from build123d import *

# Parameters (mm, degrees)
SKETCH1_R           = 25
BOSS_EXTRUDE1_DEPTH = 60
SKETCH2_R           = 25
BOSS_EXTRUDE2_DEPTH = 120.5
CUT_EXTRUDE5_DEPTH  = 60
FILLET1_R           = 12


with BuildPart() as part:
    # Sketch1 → Boss-Extrude1 (new body)
    with BuildSketch(Plane.XY):
        with BuildLine():
            Line((60, 30), (200, 30))
            Line((200, 30), (200, -30))
            Line((200, -30), (60, -30))
            ThreePointArc((60, -30), (44.188611699, -32.565835097), (30, -40))
            ThreePointArc((30, -40), (-50, 0), (30, 40))
            ThreePointArc((30, 40), (44.188611699, 32.565835097), (60, 30))
        make_face()
        Circle(SKETCH1_R, mode=Mode.SUBTRACT)
    extrude(amount=BOSS_EXTRUDE1_DEPTH)

    # Sketch2 → Boss-Extrude2 (add)
    with BuildSketch(Plane(origin=(200, 0, 0), x_dir=(0, 0, -1), z_dir=(1, 0, 0))):
        with Locations((-30, 0)):
            Circle(SKETCH2_R)
    extrude(amount=BOSS_EXTRUDE2_DEPTH)

    # Sketch8 → Cut-Extrude5 (cut)
    with BuildSketch(Plane(origin=(200, 0, 0), x_dir=(0, 0, -1), z_dir=(1, 0, 0))):
        Polygon((-60, 11.94), (-41.94, 30), (-60, 30), align=None)
        Polygon((0, 30), (-16.229667357, 30), (0, 11.94), align=None)
        Polygon((-41.94, -30), (-60, -11.94), (-60, -30), align=None)
        Polygon((0, -30), (0, -11.94), (-18.06, -30), align=None)
    extrude(amount=-CUT_EXTRUDE5_DEPTH, mode=Mode.SUBTRACT)

    # Fillet1
    fillet1_edges = [part.edges().sort_by_distance(p)[0] for p in [
        (140, -20.97, 50.97),
        (140, -20.97, 9.03),
        (140, 20.97, 8.114833678),
        (140, 20.97, 50.97),
    ]]
    fillet(fillet1_edges, radius=FILLET1_R)


solid = part.part
For this review, take the finished solid that the model builds, in its own axes (mm). A direction names the side the tool comes from. Coordinates: 2 decimals unless noted, no trailing zeros. Order: outer loops, then holes, each group sorted by start corner. A loop starts at its lowest first (then second) coordinate and runs counter-clockwise, first axis right, second up. Notation, with made-up numbers: (80, 8) - (118, 8) arc R37 cw to (118, 47) - close; hole circle Ø3 at (-11.5, 19.5). An arc over 180 degrees is marked (long way). Answer as CSV lines item,"result". Start each with the question number.
1) Add section B-B (z = 29). State the section outline as (x, y) points, then the cut area to 3 significant figures.
2) To check wall thickness, follow line 1 along Y through (x, z) = (0, 15); line 2 along X through (y, z) = (-19.5, 14); line 3 along X through (y, z) = (12, 35). State the ranges of each line that lie inside material, in increasing order. Write a range as [from, to].
3) Add section C-C (x = 0). State the section outline as (y, z) points.
4) Add section D-D (x = 186.5). State the section outline as (y, z) points, then the cut area to 3 significant figures.
5) Machinability: for faces 4 (the cylindrical face through (259, -15, 50)), 5 (the flat face through (176.34, 21.1, 8.23)), 6 (the flat face through (115, -30, 30)), which of the approach directions +Z, -Z, +X, -X, +Y, -Y give a long, thin tool a straight path to every point of the face, cutting with its end or side? Answer none if there is none.
6) Draft analysis for pull direction X (two halves, no side actions). For faces 1 (the flat face through (176.34, -20.84, 8.9)), 2 (the cylindrical face through (145.226, -22.325, 52.578)), 3 (the cylindrical face through (23.846, 7.509, 29.58)), state which applies: +X half, -X half, draft (parallel to the pull), parting line (faces both ways), or undercut.
7) Insertion check: P1, Ø12, axis at x = 40.5, y = -6.5, coming from the -Z side; P2, Ø0.9, axis at y = -29.5, z = 0.5, coming from the +X side; P3, Ø4, axis at x = 99, z = 11, coming from the -Y side; P4, Ø12, axis at x = 38.5, z = 25, coming from the -Y side. Each pin has a flat end and moves straight along its axis. Give the tip position at first contact, or say it passes through.
8) Add section A-A (y = 0). State the section outline as (x, z) points.
Result:
1,outline,"(30, -40) arc R50 cw to (60, -30) - (200, -30) - (200, -24.98) - (320.5, -24.98) - (320.5, 24.98) - (200, 24.98) - (200, 30) - (60, 30) arc R50 cw to (30, 40) arc R50 ccw (long way) to start; hole circle Ø50 at (0, 0)"
1,area,"21,200 mm^2"
2,line 1,"[-50, -25], [25, 50]"
2,line 2,"[-46.04, -15.64], [15.64, 200]"
2,line 3,"[-48.54, -21.93], [21.93, 320.5]"
3,outline,"(-50, 0) - (-25, 0) - (-25, 60) - (-50, 60) - close; (25, 0) - (50, 0) - (50, 60) - (25, 60) - close"
4,outline,"(-30, 18.06) - (-11.94, 0) - (11.94, 0) - (30, 16.23) - (30, 41.94) - (11.94, 60) - (-11.94, 60) - (-30, 41.94) - close"
4,area,"2,960 mm^2"
5,face 4,"+X"
5,face 5,"-Z, +X, +Y"
5,face 6,"+Z, -Z, +X, -Y"
6,face 1,"draft"
6,face 2,"+X half"
6,face 3,"undercut"
7,P1,"z = 0"
7,P2,"x = 140.01"
7,P3,"y = -30"
7,P4,"y = -38.24"
8,outline,"(-50, 0) - (-25, 0) - (-25, 60) - (-50, 60) - close; (25, 0) - (200, 0) - (200, 5) - (320.5, 5) - (320.5, 55) - (200, 55) - (200, 60) - (25, 60) - close"
